The model under review builds one solid part; all positions refer to its coordinate system, in mm. Round coordinates to 2 decimals unless told otherwise and drop trailing zeros. Order: outer loops, then holes, each group sorted by start corner. A loop starts at its lowest first (then second) coordinate and runs counter-clockwise, first axis right, second up.
Solid Edge part; units mm, degrees
sketch "Sketch1" plane through (0, 0, 0) normal (0, 0, 1) x (1, 0, 0)
  line L0 (-85, -92) -> (85, -92)
  line L1 (85, -92) -> (85, 92)
  line L2 (85, 92) -> (-85, 92)
  line L3 (-85, 92) -> (-85, -92)
  dimension "D1" = 85
  dimension "D2" = 85
extrude "Protrusion1" add sketch "Sketch1" along normal blind 25
sketch "Sketch2" plane through (0, -92, 12.5) normal (0, -1, 0) x (1, 0, 0)
  circle A0 centre (-62.5, -14.5) radius 16
  circle A1 centre (62.5, -14.5) radius 16
  dimension "D1" = 62.5
  dimension "D2" = 62.5
  dimension "D3" = 14.5
extrude "Cutout1" cut sketch "Sketch2" along normal mid plane 529.2958
sketch "Sketch3" plane through (0, 0, 25) normal (0, 0, 1) x (0, -1, 0)
  circle A0 centre (81, 38.75) radius 5
  circle A1 centre (-81, 38.75) radius 5
  circle A2 centre (-81, -38.75) radius 5
  circle A3 centre (81, -38.75) radius 5
  dimension "D1" = 81
  dimension "D2" = 81
extrude "ExtrudedCutout_2" cut sketch "Sketch3" along normal mid plane 360.8334
fillet "Round_1" radius 3 4 edges at (0, 92, 25) (85, 0, 25) (0, -92, 25) (-85, 0, 25)
sketch "Sketch4" plane through (0, 0, 0) normal (0, 0, -1) x (-1, 0, 0)
  line L0 (-108.1333, -70) -> (102.1809, -70)
  line L1 (102.1809, -70) -> (102.1809, 115.1165)
  line L2 (102.1809, 115.1165) -> (-108.1333, 115.1165)
  line L3 (-108.1333, 115.1165) -> (-108.1333, -70)
extrude "Cutout2" cut sketch "Sketch4" along normal mid plane 462.6347
fillet "Round_2" radius 3 4 edges at (0, -70, 25) (-84.1213, -70, 24.1213) (-85, -70, 11) (85, -70, 11)
fillet "Round1" radius 3 4 edges at (85, -92, 11) (84.1213, -91.1213, 24.1213) (-85, -92, 11) (-84.1213, -91.1213, 24.1213)
properties material "Aluminum, 6061-T6"
(1) Consider section A-A (z = 4.75). Write out the cut boundary in (x, y), and give its area (3 significant figures).
Data:
outline: (-85, -89) arc R3 ccw to (-82, -92) - (-77.01, -92) - (-77.01, -70) - (-82, -70) arc R3 ccw to (-85, -73) - close; (-47.99, -92) - (47.99, -92) - (47.99, -70) - (-47.99, -70) - close; (77.01, -92) - (82, -92) arc R3 ccw to (85, -89) - (85, -73) arc R3 ccw to (82, -70) - (77.01, -70) - close; hole circle Ø10 at (-38.75, -81); hole circle Ø10 at (38.75, -81)
area: 2,300 mm2
(2) Consider section C-C (x = 38.75). Write out the cut boundary in (y, z), and give its area (3 significant figures).
Data:
outline: (-92, 0) - (-86, 0) - (-86, 25) - (-89, 25) arc R3 ccw to (-92, 22) - close; (-76, 0) - (-70, 0) - (-70, 22) arc R3 ccw to (-73, 25) - (-76, 25) - close
area: 296 mm2
(3) Insertion check: pin 1 (5 mm diameter, centred on x = 53.5, y = -89.5, fed in from -Z); pin 2 (12 mm diameter, centred on x = -59.5, z = 5, fed in from +Y). Each pin has a flat end and moves straight along its axis. Give the tip position at first contact, or say it passes through.
Data:
pin 1: stops at z = 9.12
pin 2: passes through
(4) To check wall thickness, follow probe 1 along X at (y, z) = (-81, 19); probe 2 along X at (y, z) = (-82.25, 3.25); probe 3 along X at (y, z) = (-81, 12.5). State the ranges of each line that lie inside material, in increasing order.
Data:
probe 1: x = -85 to -43.75, -33.75 to 33.75, 43.75 to 85
probe 2: x = -85 to -77.61, -47.39 to -43.59, -33.91 to 33.91, 43.59 to 47.39, 77.61 to 85
probe 3: x = -85 to -69.26, -55.74 to -43.75, -33.75 to 33.75, 43.75 to 55.74, 69.26 to 85
(5) Draft analysis for pull direction Y (two halves, no side actions). For faces 1 (the flat face through (82, -81, 0)), 2 (the cylindrical face through (-1.15, -70.9, 24.14)), 3 (the cylindrical face through (-37.25, -85.77, 12.68)), 4 (the cylindrical face through (1.15, -91.1, 24.14)), state which applies: pulls with the +Y half, pulls with the -Y half, needs draft (parallel to the pull), parting line crosses it, or undercut.
Data:
face 1: needs draft
face 2: pulls with the +Y half
face 3: undercut
face 4: pulls with the -Y half
(6) Consider section D-D (z = 11). Write out the cut boundary in (x, y), and give its area (3 significant figures).
Data:
outline: (-85, -89) arc R3 ccw to (-82, -92) - (-71.83, -92) - (-71.83, -70) - (-82, -70) arc R3 ccw to (-85, -73) - close; (-53.17, -92) - (53.17, -92) - (53.17, -70) - (-53.17, -70) - close; (71.83, -92) - (82, -92) arc R3 ccw to (85, -89) - (85, -73) arc R3 ccw to (82, -70) - (71.83, -70) - close; hole circle Ø10 at (-38.75, -81); hole circle Ø10 at (38.75, -81)
area: 2,750 mm2
(7) Consider section B-B (y = -81). Write out the cut boundary in (x, z), and give its area (3 significant figures).
Data:
outline: (-85, 0) - (-78.37, 0) arc R16 cw to (-46.63, 0) - (-43.75, 0) - (-43.75, 25) - (-82, 25) arc R3 ccw to (-85, 22) - close; (-33.75, 0) - (33.75, 0) - (33.75, 25) - (-33.75, 25) - close; (43.75, 0) - (46.63, 0) arc R16 cw to (78.37, 0) - (85, 0) - (85, 22) arc R3 ccw to (82, 25) - (43.75, 25) - close
area: 3,070 mm2
